Build history of the part. All positions in model axes, mm. Face numbers are marked on the shaded views. A direction names the side the tool comes from. Give positions to 0.01 mm unless a question says otherwise; leave off trailing zeros. Loops run counter-clockwise (first coordinate to the right, second up) from the corner with the lowest first, then second, coordinate; pieces in that order, holes last. Notation, with made-up numbers: (-25.75, 44.5) -> (-11.75, 44.5) arc R6 cw to (-11.75, 52.5) -> close; hole circle Ø8 at (-27, 19.5). An arc over 180 degrees is marked (long way). Answer as a JSON object with one key per item and string values. Group by question number.
Q1. Band-saw the part on C-C, the plane z = -7.5. Write the cut outline in (x, y).
Q2. Drop flat-ended pins along their axis: pin 1 (5.5 mm diameter, centred on y = 10, z = -166.27, fed in from +X); pin 2 (9.5 mm diameter, centred on y = 70, z = -166.27, fed in from +X); pin 3 (7 mm diameter, centred on x = -16, y = 40, fed in from -Z); pin 4 (8 mm diameter, centred on y = 91.5, z = -50, fed in from -X). Give the stop position or say it passes through.
Q3. Band-saw the part on A-A, the plane y = 10. Write the cut outline in (x, z), plus the area to 3 significant figures.
Q4. Tool access for the marked faces 1, 2 and 3: list every direction of +Z, -Z, +X, -X, +Y, -Y with a clear straight run to the whole face (end or side of a thin tool).
Q5. Two-plate mould, pull along Z, no slides. Class the marked faces 4, 5 and 6: pulls with the +Z half, pulls with the -Z half, needs draft (parallel to the pull), parting line crosses it, or undercut.
Q6. Band-saw the part on D-D, the plane x = 22.5. Write the cut outline in (y, z), plus the area to 3 significant figures.
Q7. Wall check: probe 1 along Y at (x, z) = (-16, 17.05); probe 2 along X at (y, z) = (25, -29); probe 3 along Z at (x, y) = (-17, 7). Give the ranges that are in metal, low to high. Write a range as from..to.
Q8. Band-saw the part on B-B, the plane x = -16. Write the cut outline in (y, z), plus the area to 3 significant figures.
from build123d import *

# Parameters (mm, degrees)
EXTRUDE_1_DEPTH     = 100
FILLET_1_R          = 10
FILLET_2_R          = 3
SKETCH_2_R          = 3
CUT_EXTRUDE_1_DEPTH = 60
SKETCH_3_R          = 3
CUT_EXTRUDE_2_DEPTH = 60
FILLET_3_R          = 5
EXTRUDE_START       = 4
EXTRUDE_2_DEPTH     = 4


with BuildPart() as part:
    # Эскиз1 → Бобышка-Вытянуть1 (new body)
    with BuildSketch(Plane(origin=(0, 0, 0), x_dir=(1, 0, 0), z_dir=(0, 1, 0))):
        with BuildLine():
            Line((0, 152.272615506), (0, 176.272615506))
            Line((0, 176.272615506), (3, 176.272615506))
            Line((3, 176.272615506), (3, 155.272615506))
            ThreePointArc((3, 155.272615506), (24.600029492, 128.598973205), (57, 117.272615506))
            Line((57, 117.272615506), (57, -18.727384494))
            Line((57, -18.727384494), (-26, -18.727384494))
            Line((-26, -18.727384494), (-26, -15.727384494))
            Line((-26, -15.727384494), (54, -15.727384494))
            Line((54, -15.727384494), (54, 112.272615506))
            ThreePointArc((54, 112.272615506), (21.19671601, 124.438182118), (0, 152.272615506))
        make_face()
    extrude(amount=EXTRUDE_1_DEPTH)

    # Скругление1
    fillet_1_edges = [part.edges().sort_by_distance(p)[0] for p in [
        (57, 50, -117.272615506),
    ]]
    fillet(fillet_1_edges, radius=FILLET_1_R)

    # Скругление2
    fillet_2_edges = [part.edges().sort_by_distance(p)[0] for p in [
        (57, 50, 18.727384494),
    ]]
    fillet(fillet_2_edges, radius=FILLET_2_R)

    # Эскиз2 → Вырез-Вытянуть1 (cut)
    with BuildSketch(Plane.XY.offset(18.727384494)):
        with Locations((-16, 70)):
            Circle(SKETCH_2_R)
        with Locations((-16, 40)):
            Circle(SKETCH_2_R)
        with Locations((-16, 10)):
            Circle(SKETCH_2_R)
    extrude(amount=-CUT_EXTRUDE_1_DEPTH, mode=Mode.SUBTRACT)

    # Эскиз3 → Вырез-Вытянуть2 (cut)
    with BuildSketch(Plane(origin=(3, 0, 0), x_dir=(0, 0, -1), z_dir=(1, 0, 0))):
        with Locations((166.272615506, 10)):
            Circle(SKETCH_3_R)
        with Locations((166.272615506, 40)):
            Circle(SKETCH_3_R)
        with Locations((166.272615506, 70)):
            Circle(SKETCH_3_R)
    extrude(amount=-CUT_EXTRUDE_2_DEPTH, mode=Mode.SUBTRACT)

    # Скругление3
    fillet_3_edges = [part.edges().sort_by_distance(p)[0] for p in [
        (54, 50, -112.272615506),
    ]]
    fillet(fillet_3_edges, radius=FILLET_3_R)

    # Эскиз4 → Бобышка-Вытянуть2 (add)
    with BuildSketch(Plane(origin=(0, 100, 0), x_dir=(1, 0, 0), z_dir=(0, 1, 0)).offset(EXTRUDE_START)):
        with BuildLine():
            Line((3, 176.272615506), (0, 176.272615506))
            Line((0, 176.272615506), (0, -18.727384494))
            Line((0, -18.727384494), (54, -18.727384494))
            ThreePointArc((54, -18.727384494), (56.121320344, -17.848704838), (57, -15.727384494))
            Line((57, -15.727384494), (57, 108.468113504))
            ThreePointArc((57, 108.468113504), (54.709126709, 114.837522062), (48.886126924, 118.288629031))
            ThreePointArc((48.886126924, 118.288629031), (21.33303931, 131.060953474), (3, 155.272615506))
            Line((3, 155.272615506), (3, 176.272615506))
        make_face()
    extrude(amount=-EXTRUDE_2_DEPTH)


solid = part.part
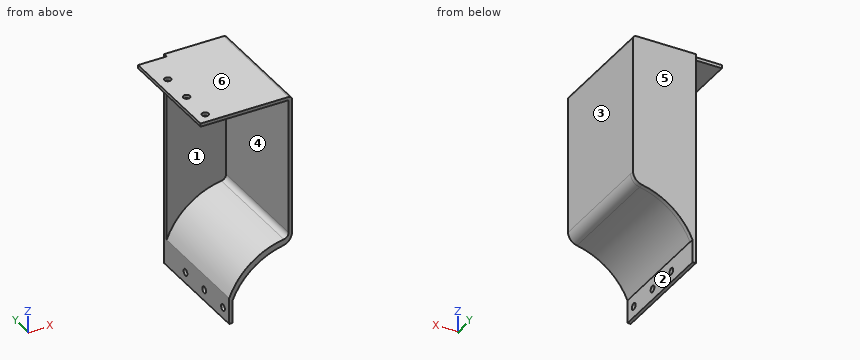
Worked answers:
{
 "1": {"outline": "(0, 100) -> (54, 100) -> (54, 0) -> (57, 0) -> (57, 104) -> (0, 104) -> close"},
 "2": {"pin 1": "through", "pin 2": "x = 3", "pin 3": "z = 15.73", "pin 4": "x = 54"},
 "3": {"outline": "(-26, 15.73) -> (-19, 15.73) -> (-19, 18.73) -> (-26, 18.73) -> close; (-13, 15.73) -> (54, 15.73) -> (54, -107.78) arc R5 cw to (49.71, -112.73) arc R62.77 ccw to (0, -152.27) -> (0, -163.27) -> (3, -163.27) -> (3, -155.27) arc R62.77 cw to (48.89, -118.29) arc R10 ccw to (57, -108.47) -> (57, 15.73) arc R3 ccw to (54, 18.73) -> (-13, 18.73) -> close; (0, -176.27) -> (3, -176.27) -> (3, -169.27) -> (0, -169.27) -> close", "area": "1,020 mm2"},
 "4": {"face 1": "-X, -Y", "face 2": "-Z, +X, +Y, -Y", "face 3": "+Z, -Z, +X, +Y, -Y"},
 "5": {"face 4": "undercut", "face 5": "needs draft", "face 6": "pulls with the +Z half"},
 "6": {"outline": "(0, -130.14) -> (104, -130.14) -> (104, 18.73) -> (0, 18.73) -> (0, 15.73) -> (100, 15.73) -> (100, -123.5) -> (0, -123.5) -> close", "area": "1,560 mm2"},
 "7": {"probe 1": "0..7, 13..37, 43..67, 73..100", "probe 2": "54..57", "probe 3": "15.73..18.73"},
 "8": {"outline": "(0, 15.73) -> (7, 15.73) -> (7, 18.73) -> (0, 18.73) -> close; (13, 15.73) -> (37, 15.73) -> (37, 18.73) -> (13, 18.73) -> close; (43, 15.73) -> (67, 15.73) -> (67, 18.73) -> (43, 18.73) -> close; (73, 15.73) -> (100, 15.73) -> (100, 18.73) -> (73, 18.73) -> close", "area": "246 mm2"}
}
